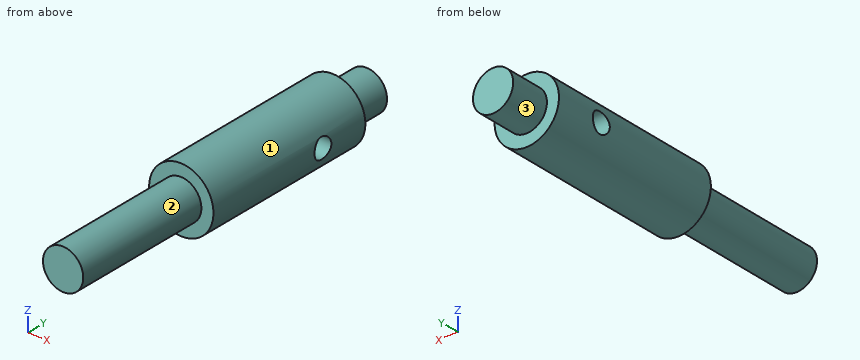
```python
from build123d import *

# Parameters (mm, degrees)
F3_R     = 2.5
F4_DEPTH = 45


with BuildPart() as f1:
    # F0 (on Top) → F1 (revolve)
    with BuildSketch(Plane.XY):
        Polygon((0, -59.698787), (0, 30.301213), (-5, 30.301213), (-5, 20.301213), (-8, 20.301213), (-8, -24.698787), (-5, -24.698787), (-5, -59.698787), align=None)
    revolve(axis=Axis((0, -14.698787, 0), (0, -1, 0)))

    # F3 (on offset) → F4 (cut)
    with BuildSketch(Plane.YZ.offset(25)):
        with Locations((7.748153, 0)):
            Circle(F3_R)
    extrude(amount=-F4_DEPTH, mode=Mode.SUBTRACT)


solid = f1.part
```
Geometry check sheet. Reference: the model listing, model coordinates, mm. Face numbers are marked on the shaded views. A direction names the side the tool comes from. Coordinates: 2 decimals unless noted, no trailing zeros. Loops run counter-clockwise (first coordinate to the right, second up) from the corner with the lowest first, then second, coordinate; pieces in that order, holes last.
Item 1: Sectioned sample at D-D, the plane z = -3.25. Record the boundary of the cut face in (x, y), then the cut area to 4 significant figures.
Item 2: Sectioned sample at C-C, the plane y = 22. Record the boundary of the cut face in (x, z).
Item 3: Sectioned sample at A-A, the plane z = 0. Record the boundary of the cut face in (x, y), then the cut area to 3 significant figures.
Item 4: Access from +Z, -Z, +X, -X, +Y, -Y to the whole of each face (thin tool, end or side, straight path). Record for the marked faces 1, 2 and 3.
Item 5: Go/stop test with flat-tipped pins: pin 1 Ø1.5 at (x, y) = (3.5, -41.5) entering from -Z; pin 2 Ø5 at (x, y) = (-2.5, -25) entering from -Z; pin 3 Ø1 at (y, z) = (-34.5, -1) entering from -X; pin 4 Ø1 at (x, z) = (-5, -3) entering from +Y. Record where each tip stops, or that it passes through.
Item 6: Thickness scan on line 1 (Y direction, x = -3.75, z = 0); line 2 (Y direction, x = -3, z = 7); line 3 (Z direction, x = 1.75, y = 8.5). Record the ranges inside material, lowest first.
Item 7: Sectioned sample at B-B, the plane x = 0. Record the boundary of the cut face in (y, z), then the cut area to 3 significant figures.
Check result:
1. outline: (-7.31, -24.7) - (-3.8, -24.7) - (-3.8, -59.7) - (3.8, -59.7) - (3.8, -24.7) - (7.31, -24.7) - (7.31, 20.3) - (3.8, 20.3) - (3.8, 30.3) - (-3.8, 30.3) - (-3.8, 20.3) - (-7.31, 20.3) - close
1. area: 1,000 mm2
2. outline: circle Ø10 at (0, 0)
3. outline: (-8, -24.7) - (-5, -24.7) - (-5, -59.7) - (5, -59.7) - (5, -24.7) - (8, -24.7) - (8, 5.25) - (-8, 5.25) - close; (-8, 10.25) - (8, 10.25) - (8, 20.3) - (5, 20.3) - (5, 30.3) - (-5, 30.3) - (-5, 20.3) - (-8, 20.3) - close
3. area: 1,090 mm2
4. face 1: +Y, -Y
4. face 2: -Y
4. face 3: +Y
5. pin 1: stops at z = -4.18
5. pin 2: stops at z = -8
5. pin 3: stops at x = -4.97
5. pin 4: stops at y = 20.3
6. line 1: y = -59.7 to 5.25, 10.25 to 30.3
6. line 2: y = -24.7 to 20.3
6. line 3: z = -7.81 to -2.38, 2.38 to 7.81
7. outline: (-59.7, -5) - (-24.7, -5) - (-24.7, -8) - (20.3, -8) - (20.3, -5) - (30.3, -5) - (30.3, 5) - (20.3, 5) - (20.3, 8) - (-24.7, 8) - (-24.7, 5) - (-59.7, 5) - close; hole circle Ø5 at (7.75, 0)
7. area: 1,150 mm2
